from build123d import *

# Parameters (mm, degrees)
BOSS_EXTRUDE1_DEPTH                            = 3.05
FILLET3_R                                      = 0.5
CSK_FOR_M3_FLAT_HEAD_MACHINE_SCREW1_AT_2_COUNT = 2
CSK_FOR_M3_FLAT_HEAD_MACHINE_SCREW1_AT_2_PITCH = 25


with BuildPart() as part:
    # Sketch1 → Boss-Extrude1 (new body)
    with BuildSketch(Plane(origin=(0, 0, 0), x_dir=(1, 0, 0), z_dir=(0, 1, 0))):
        Polygon((0, 0), (0, 43.5), (8, 43.5), (5.113248654, 38.5), (16.613248654, 38.5), (13.726497308, 43.5), (26.273502692, 43.5), (23.386751346, 38.5), (34.886751346, 38.5), (32, 43.5), (40, 43.5), (40, 0), align=None)
    extrude(amount=BOSS_EXTRUDE1_DEPTH)

    # Fillet3
    fillet3_edges = [part.edges().sort_by_distance(p)[0] for p in [
        (8, 1.525, -43.5),
        (5.113248654, 1.525, -38.5),
        (16.613248654, 1.525, -38.5),
        (13.726497308, 1.525, -43.5),
        (26.273502692, 1.525, -43.5),
        (23.386751346, 1.525, -38.5),
        (34.886751346, 1.525, -38.5),
        (32, 1.525, -43.5),
    ]]
    fillet(fillet3_edges, radius=FILLET3_R)

    # Sketch7 → CSK for M3 Flat Head Machine Screw1 (revolve, cut)
    with BuildSketch(Plane(origin=(7.5, 3.05, -4), x_dir=(0, 0, 1), z_dir=(1, 0, 0))):
        Polygon((0, 0), (0, 3.05), (1.7, 3.05), (1.7, 1.45), (3.15, 0), align=None)
    csk_for_m3_flat_head_machine_screw1 = revolve(axis=Axis((7.5, 9.4, -4), (0, -1, 0)), mode=Mode.SUBTRACT)

    # CSK for M3 Flat Head Machine Screw1 at 2: CSK for M3 Flat Head Machine Screw1 ×2
    with Locations(*[(i * CSK_FOR_M3_FLAT_HEAD_MACHINE_SCREW1_AT_2_PITCH, 0, 0) for i in range(1, CSK_FOR_M3_FLAT_HEAD_MACHINE_SCREW1_AT_2_COUNT)]):
        add(csk_for_m3_flat_head_machine_screw1, mode=Mode.SUBTRACT)


solid = part.part
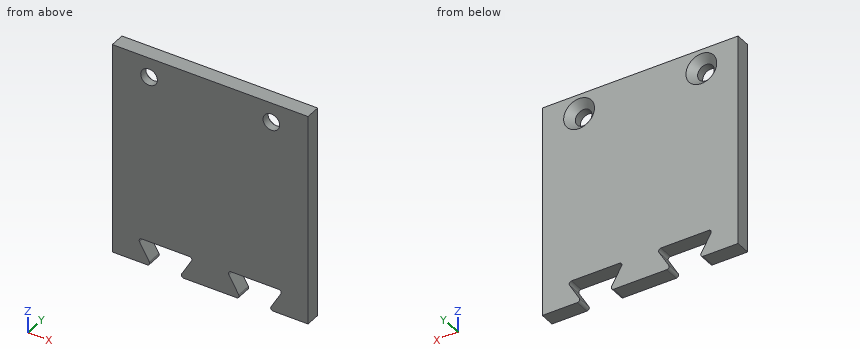
Work out the finished part from the listing and answer in its coordinate system (mm). Give positions to 0.01 mm unless a question says otherwise; leave off trailing zeros. Order: outer loops, then holes, each group sorted by start corner. A loop starts at its lowest first (then second) coordinate and runs counter-clockwise, first axis right, second up. Notation, with made-up numbers: (25.5, 27) -> (79.5, 27) arc R13 cw to (79.5, 33) -> close; hole circle Ø7 at (-30, 11). An arc over 180 degrees is marked (long way). One line per item, written item: value.
Item 1: Find section B-B, the plane z = -4. Give the vertices of the cut face in (x, y), plus the area to 3 significant figures.
Answer sheet:
outline: (0, 0) -> (5.8, 0) -> (5.8, 1.6) -> (4.35, 3.05) -> (0, 3.05) -> close; (9.2, 0) -> (30.8, 0) -> (30.8, 1.6) -> (29.35, 3.05) -> (10.65, 3.05) -> (9.2, 1.6) -> close; (34.2, 0) -> (40, 0) -> (40, 3.05) -> (35.65, 3.05) -> (34.2, 1.6) -> close
area: 97.1 mm²
Item 2: Find section C-C, the plane x = 13. Give the vertices of the cut face in (y, z).
Answer sheet:
outline: (0, -38.5) -> (3.05, -38.5) -> (3.05, 0) -> (0, 0) -> close
Item 3: Straight lines are drawn through the part: probe 1 along X at (y, z) = (1.2, -4); probe 2 along Z at (x, y) = (7.5, 0.8); probe 3 along Z at (x, y) = (11, 0.35). For each, find the intervals that lie inside material, in ascending order.
Answer sheet:
probe 1: 0 to 5.8, 9.2 to 30.8, 34.2 to 40
probe 2: -43.34 to -42.63, -38.5 to -5.7, -2.3 to 0
probe 3: -38.5 to 0
Item 4: Find section A-A, the plane y = 1.1. Give the vertices of the cut face in (x, z).
Answer sheet:
outline: (0, -43.5) -> (7.13, -43.5) arc R0.5 ccw to (7.57, -42.75) -> (5.55, -39.25) arc R0.5 cw to (5.98, -38.5) -> (15.75, -38.5) arc R0.5 cw to (16.18, -39.25) -> (14.16, -42.75) arc R0.5 ccw to (14.59, -43.5) -> (25.41, -43.5) arc R0.5 ccw to (25.84, -42.75) -> (23.82, -39.25) arc R0.5 cw to (24.25, -38.5) -> (34.02, -38.5) arc R0.5 cw to (34.45, -39.25) -> (32.43, -42.75) arc R0.5 ccw to (32.87, -43.5) -> (40, -43.5) -> (40, 0) -> (0, 0) -> close; hole circle Ø3.4 at (7.5, -4); hole circle Ø3.4 at (32.5, -4)
Item 5: Flat-ended cylindrical pins translate along their axes: P1, Ø0.9, axis at x = 29, y = 1.5, coming from the -Z side; P2, Ø2.5, axis at x = 7.5, z = -4, coming from the +Y side; P3, Ø4, axis at x = 32.5, z = -4, coming from the +Y side. Find the tip coordinate at first contact, or state that the pin passes through.
Answer sheet:
P1: z = -38.5
P2: through
P3: y = 1.9
